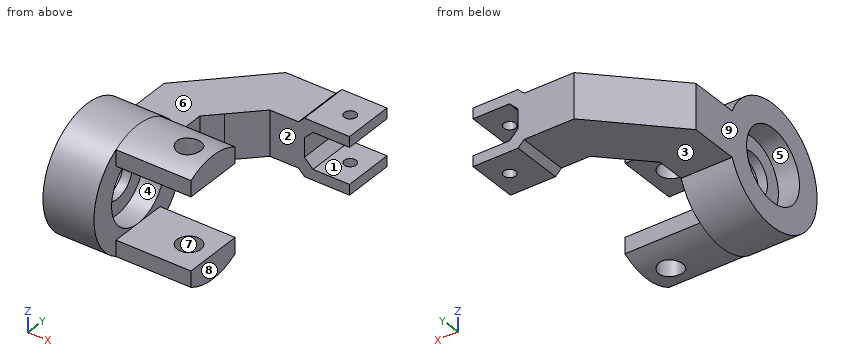
Autodesk Inventor part; units mm, degrees
ref_plane "Work Plane1" through (0, 0, 14) normal (0, 0, 1) x (1, 0, 0)
ref_plane "Work Plane2" through (0, 0, -14) normal (0, 0, 1) x (1, 0, 0)
ref_plane "YZ Plane" through (0, 0, 0) normal (1, 0, 0) x (0, 1, 0)
sketch "Sketch1" plane through (0, 0, 0) normal (0, 0, 1) x (1, 0, 0)
  line L0 (0, 7) -> (3, 7)
  line L1 (3, 7) -> (0, 7)
  line L2 (0, 7) -> (0, 12)
  line L3 (0, 12) -> (-7, 12)
  line L4 (-7, 12) -> (-7, 20)
  line L5 (-7, 20) -> (10, 20)
  line L6 (10, 20) -> (10, 12)
  line L7 (10, 12) -> (3, 12)
  line L8 (3, 12) -> (3, 7)
  line L9 (-10.4, 0) -> (13.4, 0)
  point P0 (0, 0)
  dimension "d0" = 3
  dimension "d1" = 5
  dimension "d2" = 7
  dimension "d3" = 8
  dimension "d4" = 17
  dimension "d5" = 8
  dimension "d6" = 7
revolve "Revolution1" add sketch "Sketch1" angle 360 about axis through (-10, 0, 0) along (1, 0, 0)
ref_plane "Work Plane1" through (0, 0, 14) normal (0, 0, 1) x (1, 0, 0)
ref_plane "Work Plane2" through (0, 0, -14) normal (0, 0, 1) x (1, 0, 0)
sketch "Sketch46" plane through (0, 0, 14) normal (0, 0, 1) x (1, 0, 0)
  point P0 (0, 0)
sketch "Sketch47" plane through (0, 0, 0) normal (0, 0, 1) x (1, 0, 0)
  line L0 (0, 0) -> (51.7638, 0) construction
  line L1 (-7, 41.5) -> (-7, 41.6234)
  line L2 (-7, 20) -> (10, 20)
  line L3 (-7, 20) -> (10, 20)
  line L4 (0, 0) -> (70.7107, 0) construction
  line L5 (50, 58.5) -> (50, 41.5)
  line L6 (50, 41.5) -> (30, 41.5)
  line L7 (50, 58.5) -> (30, 58.5)
  line L8 (10, -20) -> (10, 20)
  line L9 (-7, -20) -> (-7, 20)
  line L10 (-7, 20) -> (-7, 35)
  line L11 (-7, 35) -> (16.2804, 58.5)
  line L12 (16.2804, 58.5) -> (30, 58.5)
  line L13 (14.7544, 32.8045) -> (10, 28.0502)
  line L14 (10, 28.0502) -> (10, 20)
  line L15 (-7, 20) -> (10, 20)
  line L16 (14.7544, 32.8045) -> (23.4498, 41.5)
  line L17 (23.4498, 41.5) -> (30, 41.5)
  line L18 (0, 0) -> (10, 10)
extrude "Extrusion42" add sketch "Sketch47" along normal mid plane 15
sketch "Sketch54" plane through (10, 0, 0) normal (1, 0, 0) x (0, 0, -1)
  arc A0 (7.5, 18.5405) -> (-7.5, 18.5405) centre (0, 0) ccw
  line L0 (-7.5, 20) -> (0, 20)
  line L1 (7.5, 20) -> (-7.5, 20)
  line L2 (-7.5, 20) -> (-7.5, 18.5405)
  line L3 (7.5, 20) -> (7.5, 18.5405)
  circle A1 centre (0, 0) radius 20
extrude "Extrusion48" add sketch "Sketch54" against normal up to surface (17 mm away) contours A0 L1 L3 | A0 L2 L0
sketch "Sketch55" plane through (10, 18.5405, 7.5) normal (1, 0, 0) x (0, 0, -1)
  line L0 (19.5, -8.5405) -> (19.5, -28.5405)
  line L1 (19.5, -8.5405) -> (24.8205, -8.5405)
  line L2 (19.5, -28.5405) -> (24.8205, -28.5405)
  arc A0 (0, 0) -> (15, 0) centre (7.5, -18.5405) ccw
  line L3 (-4.5, -8.5405) -> (-4.5, -28.5405)
  line L4 (-4.5, -8.5405) -> (-9.8205, -8.5405)
  line L5 (-4.5, -28.5405) -> (-9.8205, -28.5405)
  arc A1 (24.8205, -28.5405) -> (24.8205, -8.5405) centre (7.5, -18.5405) ccw
  arc A2 (-9.8205, -8.5405) -> (-9.8205, -28.5405) centre (7.5, -18.5405) ccw
  point P0 (19.5, -18.5405)
extrude "Extrusion49" add sketch "Sketch55" along normal blind 25
sketch "Sketch56" plane through (10, -10, 12) normal (0, 0, -1) x (-1, 0, 0)
  circle A0 centre (-17, 10) radius 4
  line L0 (-25, 0) -> (-25, 20)
  point P0 (10, 10)
  point P1 (-25, 10)
  dimension "d298" = 8
  dimension "d299" = 8
extrude "Extrusion50" cut sketch "Sketch56" along normal through all both and the other way through all
sketch "Sketch57" plane through (23.4498, 41.5, 7.5) normal (0, -1, 0) x (1, 0, 0)
  line L0 (26.5502, -15) -> (26.5502, 0)
  line L1 (26.5502, -13.5) -> (11.5502, -13.5)
  line L2 (11.5502, -13.5) -> (11.5502, -1.5)
  line L3 (11.5502, -1.5) -> (26.5502, -1.5)
  line L4 (26.5502, -1.5) -> (26.5502, -13.5)
  point P0 (-23.4498, -7.5)
  point P1 (26.5502, -7.5)
  point P2 (11.5502, -7.5)
  dimension "d302" = 15
  dimension "d303" = 12
  dimension "d304" = 0
extrude "Extrusion51" cut sketch "Sketch57" against normal through all
sketch "Sketch59" plane through (0, 0, -7.5) normal (0, 0, -1) x (-1, 0, 0)
  point P0 (0, 0)
sketch "Sketch60" plane through (0, 0, -7.5) normal (0, 0, -1) x (-1, 0, 0)
  point P0 (0, 0)
sketch "Sketch62" plane through (16.2804, 58.5, -7.5) normal (0, 1, 0) x (1, 0, 0)
  line L0 (18.7196, -1.5) -> (33.7196, -1.5)
  line L1 (0, 0) -> (33.7196, 0)
  line L2 (18.7196, 0) -> (33.7196, 0)
  line L3 (33.7196, 0) -> (33.7196, 2)
  line L4 (33.7196, 2) -> (18.7196, 2)
  line L5 (33.7196, -15) -> (0, -15)
  line L6 (18.7196, -15) -> (33.7196, -15)
  line L7 (33.7196, -15) -> (33.7196, -17)
  line L8 (33.7196, -17) -> (18.7196, -17)
  line L9 (18.7196, 2) -> (16.7196, 0)
  line L10 (33.7196, 0) -> (7.1694, 0)
  line L11 (18.7196, 2) -> (21.548, 2) construction
  line L12 (18.7196, 0) -> (16.7196, 0)
  line L13 (18.7196, -17) -> (16.7196, -15)
  line L14 (18.7196, -15) -> (16.7196, -15)
  point P0 (-16.2804, -7.5)
  point P1 (16.7196, 0)
  dimension "d318" = 2
  dimension "d319" = 2
  dimension "d322" = 135
extrude "Extrusion53" add sketch "Sketch62" against normal up to surface (17 mm away)
sketch "Sketch63" plane through (50, 41.5, 6) normal (0, 0, -1) x (-1, 0, 0)
  circle A0 centre (6, 8.5) radius 2
  line L0 (0, 0) -> (0, 17)
  point P0 (50, -41.5)
  dimension "d323" = 4
  dimension "d324" = 6
extrude "Extrusion54" cut sketch "Sketch63" along normal through all both and the other way through all
sketch "Sketch64" plane through (16.2804, 58.5, 7.5) normal (0, 1, 0) x (1, 0, 0)
  line L0 (18.7196, 1.5) -> (33.7196, 1.5)
  line L1 (21.548, 1.5) -> (18.7196, 4.3284)
  line L2 (21.548, 1.5) -> (25.548, 1.5) construction
  line L3 (18.7196, 1.5) -> (18.7196, 13.5)
  line L4 (21.548, 1.5) -> (18.7196, 1.5)
  line L5 (18.7196, 13.5) -> (33.7196, 13.5)
  line L6 (21.548, 13.5) -> (18.7196, 10.6716)
  line L7 (21.548, 13.5) -> (25.548, 13.5) construction
  line L8 (18.7196, 13.5) -> (18.7196, 1.5)
  line L9 (18.7196, 10.6716) -> (18.7196, 13.5)
  line L10 (18.7196, 13.5) -> (21.548, 13.5)
  line L11 (18.7196, 1.5) -> (18.7196, 4.3284)
  point P0 (-16.2804, 7.5)
  point P1 (18.7196, 4.3284)
  dimension "d327" = 4
  dimension "d328" = 135
  dimension "d329" = 0
  dimension "d330" = 135
  dimension "d331" = 4
  dimension "d332" = 0
extrude "Extrusion55" add sketch "Sketch64" against normal up to surface (17 mm away)
properties part number "Wheel hub left ver 2"
The model under review builds one solid part; all positions refer to its coordinate system, in mm. Face numbers are marked on the shaded views. A direction names the side the tool comes from. Round coordinates to 2 decimals unless told otherwise and drop trailing zeros. Loops run counter-clockwise (first coordinate to the right, second up) from the corner with the lowest first, then second, coordinate; pieces in that order, holes last. Notation, with made-up numbers: (-1.5, 15.5) -> (14.5, 15.5) arc R23 cw to (14.5, 23.5) -> close; hole circle Ø5 at (-39, 82.25). An arc over 180 degrees is marked (long way). Write item = value, one per line. Start each with the question number.
Item 1: Mouldability with a two-part tool opening along X and no side actions: class the marked faces 6, 7, 8 and 9 as released by +X, released by -X, zero draft, split by the parting line, or undercut.
Item 2: To check wall thickness, follow L1, parallel to Y at x = 44, z = -7; L2, parallel to X at y = 0, z = -18; L3, parallel to Y at x = 27, z = 14. State the ranges of each line that lie inside material, in increasing order.
Item 3: Take a section at A-A on x = 44. Give the boundary of the cut face in (y, z), plus the area to 3 significant figures.
Item 4: Insertion check: pin 1 (6 mm diameter, centred on x = 18.5, y = -3.5, fed in from -Z); pin 2 (6 mm diameter, centred on x = 8, y = 48, fed in from +Z); pin 3 (7 mm diameter, centred on y = 47.5, z = 0.5, fed in from +X). Each pin has a flat end and moves straight along its axis. Give the tip position at first contact, or say it passes through.
Item 5: Take a section at C-C on y = -3. Give the boundary of the cut face in (x, z).
Item 6: Take a section at B-B on z = 0. Give the boundary of the cut face in (x, y).
Item 7: Take a section at D-D on x = 27. Give the boundary of the cut face in (y, z), plus the area to 3 significant figures.
Item 8: For the marked faces 1, 2, 3, 4 and 5, list the 3-axis set-ups (+Z, -Z, +X, -X, +Y, -Y) from which the entire face can be reached by the end or side of a thin tool; tool diameter is ignored.
Result:
q1.face_6 = zero draft
q1.face_7 = undercut
q1.face_8 = released by +X
q1.face_9 = released by -X
q2.L1 = 41.5 to 48, 52 to 58.5
q2.L2 = -7 to 23, 31 to 35
q2.L3 = -10 to -4, 4 to 10
q3.outline = (41.5, -9.5) -> (48, -9.5) -> (48, -6) -> (41.5, -6) -> close; (41.5, 6) -> (48, 6) -> (48, 9.5) -> (41.5, 9.5) -> close; (52, -9.5) -> (58.5, -9.5) -> (58.5, -6) -> (52, -6) -> close; (52, 6) -> (58.5, 6) -> (58.5, 9.5) -> (52, 9.5) -> close
q3.area = 91.0 mm²
q4.pin_1 = -19.99
q4.pin_2 = 7.5
q4.pin_3 = 35.83
q5.outline = (-7, -19.77) -> (24.35, -19.77) -> (24.35, -12) -> (10, -12) -> (10, -11.62) -> (3, -11.62) -> (3, -6.32) -> (0, -6.32) -> (0, -11.62) -> (-7, -11.62) -> close; (-7, 11.62) -> (0, 11.62) -> (0, 6.32) -> (3, 6.32) -> (3, 11.62) -> (10, 11.62) -> (10, 12) -> (24.35, 12) -> (24.35, 19.77) -> (-7, 19.77) -> close; (29.65, -19.77) -> (35, -19.77) -> (35, -12) -> (29.65, -12) -> close; (29.65, 12) -> (35, 12) -> (35, 19.77) -> (29.65, 19.77) -> close
q6.outline = (-7, -20) -> (10, -20) -> (10, -12) -> (3, -12) -> (3, -7) -> (0, -7) -> (0, -12) -> (-7, -12) -> close; (-7, 12) -> (0, 12) -> (0, 7) -> (3, 7) -> (3, 12) -> (10, 12) -> (10, 28.05) -> (14.75, 32.8) -> (23.45, 41.5) -> (35, 41.5) -> (35, 58.5) -> (16.28, 58.5) -> (-7, 35) -> close
q7.outline = (-10, -17.32) arc R20 ccw to (-4, -19.6) -> (-4, -12) -> (-10, -12) -> close; (-10, 12) -> (-4, 12) -> (-4, 19.6) arc R20 ccw to (-10, 17.32) -> close; (4, -19.6) arc R20 ccw to (10, -17.32) -> (10, -12) -> (4, -12) -> close; (4, 12) -> (10, 12) -> (10, 17.32) arc R20 ccw to (4, 19.6) -> close; (41.5, -7.5) -> (58.5, -7.5) -> (58.5, 7.5) -> (41.5, 7.5) -> close
q7.area = 414 mm²
q8.face_1 = +X, +Y, -Y
q8.face_2 = +Z, -Z, +X, -Y
q8.face_3 = -Z, -X, +Y
q8.face_4 = +X
q8.face_5 = -X
